Check sheet for the modelled part. Datum: model origin and axes. Units: mm. Round coordinates to 2 decimals unless told otherwise and drop trailing zeros. One line per item, written item: value.
from build123d import *

# Parameters (mm, degrees)
F0_R     = 3
F0_R_2   = 2.5
F1_DEPTH = 973
F2_R     = 2
F3_R     = 7
F5_DEPTH = 30


# Not quite as in the source:
# - a feature names something its author has since deleted; it is built from what else it names


with BuildPart() as f1:
    # F0 (on Top) → F1 (new body)
    with BuildSketch(Plane.XY):
        with BuildLine():
            Line((18.15, -15), (30, -15))
            Line((30, -15), (30, -3.15))
            Line((30, -3.15), (27.5, -3.15))
            Line((27.5, -3.15), (27.5, -5.15))
            Line((27.5, -5.15), (21.5477069044, -5.15))
            ThreePointArc((21.5477069044, -5.15), (19.5, 0), (21.5477069044, 5.15))
            Line((21.5477069044, 5.15), (27.5, 5.15))
            Line((27.5, 5.15), (27.5, 3.15))
            Line((27.5, 3.15), (30, 3.15))
            Line((30, 3.15), (30, 15))
            Line((30, 15), (18.15, 15))
            Line((18.15, 15), (18.15, 12.5))
            Line((18.15, 12.5), (20.15, 12.5))
            Line((20.15, 12.5), (20.15, 6.5477069044))
            ThreePointArc((20.15, 6.5477069044), (15, 4.5), (9.85, 6.5477069044))
            Line((9.85, 6.5477069044), (9.85, 12.5))
            Line((9.85, 12.5), (11.85, 12.5))
            Line((11.85, 12.5), (11.85, 15))
            Line((11.85, 15), (-11.85, 15))
            Line((-11.85, 15), (-11.85, 12.5))
            Line((-11.85, 12.5), (-9.85, 12.5))
            Line((-9.85, 12.5), (-9.85, 6.5477069044))
            ThreePointArc((-9.85, 6.5477069044), (-15, 4.5), (-20.15, 6.5477069044))
            Line((-20.15, 6.5477069044), (-20.15, 12.5))
            Line((-20.15, 12.5), (-18.15, 12.5))
            Line((-18.15, 12.5), (-18.15, 15))
            Line((-18.15, 15), (-30, 15))
            Line((-30, 15), (-30, 3.15))
            Line((-30, 3.15), (-27.5, 3.15))
            Line((-27.5, 3.15), (-27.5, 5.15))
            Line((-27.5, 5.15), (-21.5477069044, 5.15))
            ThreePointArc((-21.5477069044, 5.15), (-19.5, 0), (-21.5477069044, -5.15))
            Line((-21.5477069044, -5.15), (-27.5, -5.15))
            Line((-27.5, -5.15), (-27.5, -3.15))
            Line((-27.5, -3.15), (-30, -3.15))
            Line((-30, -3.15), (-30, -15))
            Line((-30, -15), (-18.15, -15))
            Line((-18.15, -15), (-18.15, -12.5))
            Line((-18.15, -12.5), (-20.15, -12.5))
            Line((-20.15, -12.5), (-20.15, -6.5477069044))
            ThreePointArc((-20.15, -6.5477069044), (-15, -4.5), (-9.85, -6.5477069044))
            Line((-9.85, -6.5477069044), (-9.85, -12.5))
            Line((-9.85, -12.5), (-11.85, -12.5))
            Line((-11.85, -12.5), (-11.85, -15))
            Line((-11.85, -15), (11.85, -15))
            Line((11.85, -15), (11.85, -12.5))
            Line((11.85, -12.5), (9.85, -12.5))
            Line((9.85, -12.5), (9.85, -6.5477069044))
            ThreePointArc((9.85, -6.5477069044), (15, -4.5), (20.15, -6.5477069044))
            Line((20.15, -6.5477069044), (20.15, -12.5))
            Line((20.15, -12.5), (18.15, -12.5))
            Line((18.15, -12.5), (18.15, -15))
        make_face()
        with Locations((-25, -10)):
            Circle(F0_R, mode=Mode.SUBTRACT)
        with Locations((25, -10)):
            Circle(F0_R, mode=Mode.SUBTRACT)
        with Locations((-15, 0)):
            Circle(F0_R_2, mode=Mode.SUBTRACT)
        with Locations((-25, 10)):
            Circle(F0_R, mode=Mode.SUBTRACT)
        Polygon((-7, 7), (-7, 12.5), (0, 12.5), (7, 12.5), (7, 7), (10, 0), (7, -7), (7, -12.5), (0, -12.5), (-7, -12.5), (-7, -7), (-10, 0), align=None, mode=Mode.SUBTRACT)
        with Locations((15, 0)):
            Circle(F0_R_2, mode=Mode.SUBTRACT)
        with Locations((25, 10)):
            Circle(F0_R, mode=Mode.SUBTRACT)
    extrude(amount=F1_DEPTH)

    # F2
    f2_edges = [f1.edges().sort_by_distance(p)[0] for p in [
        (-7, 12.5, 486.5),
        (7, 12.5, 486.5),
    ]]
    fillet(f2_edges, radius=F2_R)

    # F3
    f3_edges = [f1.edges().sort_by_distance(p)[0] for p in [
        (-7, 7, 486.5),
        (-10, 0, 486.5),
        (7, 7, 486.5),
        (10, 0, 486.5),
    ]]
    fillet(f3_edges, radius=F3_R)

    # F4 (on Right) → F5 (cut, symmetric)
    with BuildSketch(Plane.YZ):
        Polygon((15, 30), (-15, 0), (15, 0), align=None)
        Polygon((15, 973), (-15, 973), (15, 943), align=None)
    extrude(amount=F5_DEPTH, both=True, mode=Mode.SUBTRACT)


solid = f1.part
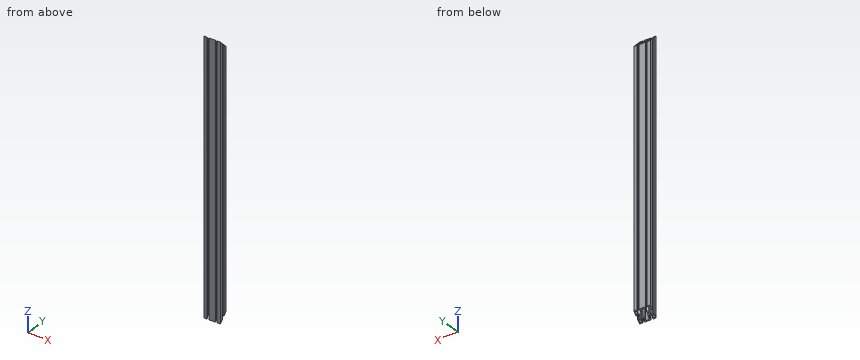
Q1. Sectioned sample at A-A on z = 569.5. State how many separate pieces and enclosed holes the cut face has, and give its area (3 significant figures).
Completed:
separate pieces: 1
enclosed holes: 7
area: 710 mm^2
Q2. Depth check by flat-ended pin: P1, Ø3, axis at x = 9.5, y = 2, coming from the +Z side; P2, Ø3, axis at x = 12, y = 4.5, coming from the -Z side; P3, Ø10, axis at x = 18.5, y = -4, coming from the -Z side; P4, Ø5, axis at x = 17, y = 8.5, coming from the -Z side. Enter the tip coordinate at first touch or a pass-through.
Completed:
P1: z = 957.5
P2: z = 18
P3: z = 6.28
P4: through
Q3. Scan lines: line 1 (X direction, y = 0.5, z = 356.5); line 2 (Y direction, x = -26, z = 69.5); line 3 (Y direction, x = -25, z = 290.5). Record each from-to range of solid material in increasing order. Write a range as [from, to].
Completed:
line 1: [-19.52, -17.45], [-12.55, -9.37], [9.37, 12.55], [17.45, 19.52]
line 2: [-15, -12.83], [-7.17, -5.15], [5.15, 7.17], [12.83, 15]
line 3: [-15, -13], [-7, -5.15], [5.15, 7], [13, 15]
